Part model, mm, in its own coordinate system. A direction names the side the tool comes from. Give positions to 0.01 mm unless a question says otherwise; leave off trailing zeros. Write each loop counter-clockwise with the first axis right and the second up, starting at its lowest first coordinate (ties: lowest second). Pieces come first, ordered by that corner, then holes. Notation, with made-up numbers: (80, 88.5) - (129, 88.5) arc R20 ccw to (129, 100.5) - close; hole circle Ø1 at (53, 63.5). An arc over 180 degrees is marked (long way). Answer as a JSON object with one key per item and string values. Group by question number.
```python
from build123d import *

# Parameters (mm, degrees)
SIDE_LIP_MAIN_SECTION_W          = 6
SIDE_LIP_MAIN_SECTION_H          = 108
SIDE_LIP_DEPTH                   = 5
VERTICAL_FIN_CUTS_DEPTH          = 2.6
SKETCH4_W                        = 3.5
SKETCH4_H                        = 108
DESCENDER_DEPTH                  = 4.5
SKETCH5_W                        = 108
SKETCH5_H                        = 2.5
PCB_BASE_DEPTH                   = 4
LOWER_CAP_DEPTH                  = 2
SKETCH9_W                        = 3
SKETCH9_H                        = 2.5
AL_BAR_CUT_DEPTH                 = 4
SKETCH10_W                       = 12.653731328
SKETCH10_H                       = 2.5
SKETCH10_W_2                     = 10.7
SUPPORT_TABS_DEPTH               = 8
BOLT_HOLES_REACH                 = 4.5
SKETCH11_R                       = 1.65
AL_BAR_ENCLOSURE_DEPTH           = 7.5
AL_BAR_BASE_DEPTH                = 2
FILLET1_R                        = 2
SKETCH16_W                       = 10
SKETCH16_H                       = 0.5
REDUCE_SIDE_SUPPORT_HEIGHT_DEPTH = 111
SIT_FLAT_DEPTH                   = 111
SKETCH19_W                       = 110
SKETCH19_H                       = 1
LOWER_TOP_DEPTH                  = 19


with BuildPart() as part:
    # Side lip main section → Side lip (new body)
    with BuildSketch(Plane(origin=(0, 0, 0), x_dir=(1, 0, 0), z_dir=(0, 1, 0))):
        with Locations((3, -54)):
            Rectangle(SIDE_LIP_MAIN_SECTION_W, SIDE_LIP_MAIN_SECTION_H)
    extrude(amount=-SIDE_LIP_DEPTH)

    # Sketch2 → Vertical fin cuts (cut)
    with BuildSketch(Plane.ZY):
        Polygon((102, 0), (103.246640014, -5), (101.70071957, -5), (100.454079556, 0), align=None)
        Polygon((75, 0), (76.246640014, -5), (74.70071957, -5), (73.454079556, 0), align=None)
        Polygon((48, 0), (49.246640014, -5), (47.70071957, -5), (46.454079556, 0), align=None)
        Polygon((21, 0), (22.246640014, -5), (20.70071957, -5), (19.454079556, 0), align=None)
    extrude(amount=-VERTICAL_FIN_CUTS_DEPTH, mode=Mode.SUBTRACT)

    # Sketch4 → Descender (add)
    with BuildSketch(Plane.XZ.offset(5)):
        with Locations((4.25, 54)):
            Rectangle(SKETCH4_W, SKETCH4_H)
    extrude(amount=DESCENDER_DEPTH)

    # Sketch5 → PCB base (add)
    with BuildSketch(Plane(origin=(6, 0, 0), x_dir=(0, 0, -1), z_dir=(1, 0, 0))):
        with Locations((-54, -8.25)):
            Rectangle(SKETCH5_W, SKETCH5_H)
    extrude(amount=PCB_BASE_DEPTH)

    # Sketch8 → Lower cap (add)
    with BuildSketch(Plane.XY.offset(108)):
        Polygon((6, 0), (10, 0), (10, -7), (10, -9.5), (2.5, -9.5), (2.5, -5), (0, -5), (0, 0), align=None)
    extrude(amount=LOWER_CAP_DEPTH)

    # Sketch9 → Al bar cut (cut)
    with BuildSketch(Plane(origin=(10, 0, 0), x_dir=(0, 0, -1), z_dir=(1, 0, 0))):
        with Locations((-12.2, -8.25)):
            Rectangle(SKETCH9_W, SKETCH9_H)
    extrude(amount=-AL_BAR_CUT_DEPTH, mode=Mode.SUBTRACT)

    # Sketch10 → Support tabs (add)
    with BuildSketch(Plane(origin=(10, 0, 0), x_dir=(0, 0, -1), z_dir=(1, 0, 0))):
        with Locations((-101.673134336, -8.25)):
            Rectangle(SKETCH10_W, SKETCH10_H)
        with Locations((-5.35, -8.25)):
            Rectangle(SKETCH10_W_2, SKETCH10_H)
    extrude(amount=SUPPORT_TABS_DEPTH)

    # Sketch11 → Bolt holes (cut, up to next)
    with BuildSketch(Plane(origin=(0, -7, 0), x_dir=(1, 0, 0), z_dir=(0, 1, 0)), mode=Mode.PRIVATE) as bolt_holes_sk1:
        with Locations((13, -5)):
            Circle(SKETCH11_R)
    bolt_holes_tool1 = extrude(bolt_holes_sk1.sketch, amount=-BOLT_HOLES_REACH, mode=Mode.PRIVATE) & part.part
    add(bolt_holes_tool1.solids().sort_by_distance((13, -7, 5))[0], mode=Mode.SUBTRACT)
    # Sketch11 → Bolt holes (cut, up to next)
    with BuildSketch(Plane(origin=(0, -7, 0), x_dir=(1, 0, 0), z_dir=(0, 1, 0)), mode=Mode.PRIVATE) as bolt_holes_sk2:
        with Locations((13, -101)):
            Circle(SKETCH11_R)
    bolt_holes_tool2 = extrude(bolt_holes_sk2.sketch, amount=-BOLT_HOLES_REACH, mode=Mode.PRIVATE) & part.part
    add(bolt_holes_tool2.solids().sort_by_distance((13, -7, 101))[0], mode=Mode.SUBTRACT)

    # Sketch12 → Al bar enclosure (add)
    with BuildSketch(Plane.XZ.offset(9.5)):
        Polygon((6, 10.7), (18, 10.7), (18, 8.7), (4, 8.7), (4, 15.7), (10, 15.7), (10, 13.7), (6, 13.7), align=None)
    extrude(amount=AL_BAR_ENCLOSURE_DEPTH)

    # Sketch13 → Al bar base (add)
    with BuildSketch(Plane.XZ.offset(17)):
        Polygon((10, 15.7), (4, 15.7), (4, 8.7), (18, 8.7), (18, 10.7), align=None)
    extrude(amount=AL_BAR_BASE_DEPTH)

    # Fillet1
    fillet1_edges = [part.edges().sort_by_distance(p)[0] for p in [
        (18, -8.25, 108),
        (18, -8.25, 95.346268672),
        (18, -8.25, 0),
        (4, -14.25, 15.7),
        (4, -14.25, 8.7),
    ]]
    fillet(fillet1_edges, radius=FILLET1_R)

    # Sketch16 → Reduce side support height (cut, through all)
    with BuildSketch(Plane.XY.offset(110)):
        with Locations((5, -0.25)):
            Rectangle(SKETCH16_W, SKETCH16_H)
    extrude(amount=-REDUCE_SIDE_SUPPORT_HEIGHT_DEPTH, mode=Mode.SUBTRACT)

    # Sketch17 → Sit flat! (cut, through all)
    with BuildSketch(Plane.XY.offset(110)):
        Polygon((2.5, -5), (2.7, -5), (3, -9.5), (2.5, -9.5), align=None)
    extrude(amount=-SIT_FLAT_DEPTH, mode=Mode.SUBTRACT)

    # Sketch19 → Lower top (cut, through all)
    with BuildSketch(Plane.ZY):
        with Locations((55, -1)):
            Rectangle(SKETCH19_W, SKETCH19_H)
    extrude(amount=-LOWER_TOP_DEPTH, mode=Mode.SUBTRACT)


solid = part.part
```
1) Saw through at C-C (y = -13.75). List the corners of the cut face in (x, z).
2) Drill centre lines: line 1 along Z through (x, y) = (13, -8.6); line 2 along Z through (x, y) = (14.75, -8.75); line 3 along Y through (x, z) = (5.5, 63). Where is each one in solid material? Low to high. Write a range as from..to.
3) Saw through at B-B (x = 13). List the corners of the cut face in (y, z) (3 decimals).
4) Saw through at A-A (z = 71). List the corners of the cut face in (x, y).
5) Drop flat-ended pins along their axis: P1, Ø1.5, axis at x = 6, y = -12.5, coming from the -Z side; P2, Ø5, axis at x = 11, z = 84.5, coming from the -Y side; P3, Ø5.5, axis at x = 11.5, z = 14, coming from the +Y side. Give the stop position or say it passes through.
6) Which spindle directions (+Z, -Z, +X, -X, +Y, -Y) get a long thin tool onto all of the face, cutting with end or side? Do faces 4 (the cylindrical face through (17.4, -8.23, 95.92)), 5 (the flat face through (13, -8, 108)), 6 (the flat face through (12, -12, 10.7)), 7 (the flat face through (1.28, -3.27, 74.27)). Say none if no direction does.
7) Saw through at D-D (x = 7). List the corners of the cut face in (y, z).
8) Two-plate mould, pull along Z, no slides. Class faces 1 (the flat face through (9, -19, 11)), 2 (the flat face through (8, -4, 108)), 3 (the flat face through (1.28, -3.27, 20.27)): +Z half, -Z half, draft (parallel to the pull), parting line (faces both ways), or undercut.
Checks:
{
 "1": {"outline": "(4, 10.7) arc R2 ccw to (6, 8.7) - (18, 8.7) - (18, 10.7) - (6, 10.7) - (6, 13.7) - (10, 13.7) - (10, 15.7) - (6, 15.7) arc R2 ccw to (4, 13.7) - close"},
 "2": {"line 1": "0..3.35, 6.65..10.7, 95.35..99.35, 102.65..108", "line 2": "0..10.7, 95.35..108", "line 3": "-9.5..-1.5"},
 "3": {"outline": "(-19, 8.7) - (-9.5, 8.7) - (-9.5, 6.65) - (-7, 6.65) - (-7, 10.7) - (-17, 10.7) - (-17, 13.825) - (-19, 13.825) - close; (-9.5, 0) - (-7, 0) - (-7, 3.35) - (-9.5, 3.35) - close; (-9.5, 95.346) - (-7, 95.346) - (-7, 99.35) - (-9.5, 99.35) - close; (-9.5, 102.65) - (-7, 102.65) - (-7, 108) - (-9.5, 108) - close"},
 "4": {"outline": "(0, -5) - (2.7, -5) - (3, -9.5) - (10, -9.5) - (10, -7) - (6, -7) - (6, -1.5) - (0, -1.5) - close"},
 "5": {"P1": "z = 8.7", "P2": "y = -9.5", "P3": "y = -7"},
 "6": {"face 4": "+X, +Y, -Y", "face 5": "+Z, +X, +Y, -Y", "face 6": "+X, +Y", "face 7": "-X, +Y"},
 "7": {"outline": "(-19, 8.7) - (-9.5, 8.7) - (-9.5, 0) - (-7, 0) - (-7, 10.7) - (-17, 10.7) - (-17, 13.7) - (-7, 13.7) - (-7, 108) - (-1.5, 108) - (-1.5, 110) - (-9.5, 110) - (-9.5, 15.7) - (-19, 15.7) - close"},
 "8": {"face 1": "draft", "face 2": "-Z half", "face 3": "undercut"}
}
